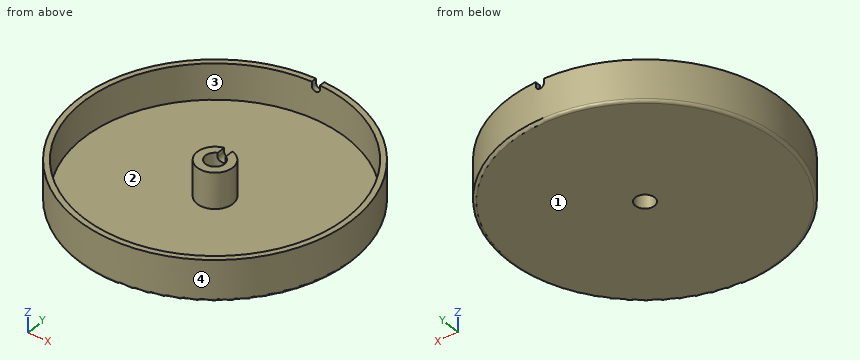
from build123d import *

# Parameters (mm, degrees)
F0_R     = 48
F0_R_2   = 6.5
F1_DEPTH = 2
F0_R_3   = 50
F0_R_4   = 3.5
F2_DEPTH = 15
F4_DEPTH = 70
F5_R     = 1


with BuildPart() as f1:
    # F0 (on Top) → F1 (new body)
    with BuildSketch(Plane.XY):
        Circle(F0_R)
        Circle(F0_R_2, mode=Mode.SUBTRACT)
    extrude(amount=F1_DEPTH)

    # F0 (on Top) → F2 (join)
    with BuildSketch(Plane.XY):
        Circle(F0_R_3)
        Circle(F0_R, mode=Mode.SUBTRACT)
        Circle(F0_R_2)
        Circle(F0_R_4, mode=Mode.SUBTRACT)
    extrude(amount=F2_DEPTH)

    # F3 (on Front) → F4 (cut)
    with BuildSketch(Plane.XZ):
        with BuildLine():
            ThreePointArc((-1.5, 13.5), (0, 15), (1.5, 13.5))
            Line((1.5, 13.5), (1.5, 16.5))
            Line((1.5, 16.5), (-1.5, 16.5))
            Line((-1.5, 16.5), (-1.5, 13.5))
        make_face()
        with BuildLine():
            Line((-1.5, 13.5), (1.5, 13.5))
            ThreePointArc((1.5, 13.5), (0, 15), (-1.5, 13.5))
        make_face()
        with BuildLine():
            ThreePointArc((-1.5, 13.5), (0, 12), (1.5, 13.5))
            Line((1.5, 13.5), (-1.5, 13.5))
        make_face()
    extrude(amount=-F4_DEPTH, mode=Mode.SUBTRACT)

    # F5
    f5_edges = [f1.edges().sort_by_distance(p)[0] for p in [
        (-50, 0, 0),
    ]]
    fillet(f5_edges, radius=F5_R)


solid = f1.part
Read the model definition and answer for the solid it produces. Units are mm, in the model's axes. Face numbers are marked on the shaded views. Coordinates: 2 decimals unless noted, no trailing zeros. Order: outer loops, then holes, each group sorted by start corner. A loop starts at its lowest first (then second) coordinate and runs counter-clockwise, first axis right, second up. Notation, with made-up numbers: M 61,-26.5 L 75,-26.5 A25 ccw 75,12.5 Z; hole C 43.5,-12.5 d1. An arc over 180 degrees is marked long. Put each result on its own line as item: value. Start each with the question number.
Item 1: The mould has two halves that part along Y. Classify the marked faces 1, 2, 3 and 4: +Y half, -Y half, draft (parallel to the pull), parting line (faces both ways), or undercut.
Item 2: Section C-C, the plane z = 10.25 is taken. Determine the outline of the cut face in (x, y).
Item 3: Given pin 1 Ø1.2 at (y, z) = (5, 14.5) entering from +X; pin 2 Ø2 at (x, z) = (14, 12.5) entering from +Y; pin 3 Ø1.5 at (x, y) = (-20.5, -1.5) entering from +Z, each flat-ended and moving along its own axis, determine where each tip first touches the part or whether it passes through.
Item 4: Section A-A, the plane x = 0 is taken. Determine the outline of the cut face in (y, z).
Item 5: Section B-B, the plane y = 0 is taken. Determine the outline of the cut face in (x, z), plus the area to 3 significant figures.
Item 6: Consider probe 1 along X at (y, z) = (0, 3.25); probe 2 along X at (y, z) = (-3, 7.75). Determine where each line is inside the solid, lowest interval first. Write a range as [from, to].
Computed:
1. face 1: draft
1. face 2: undercut
1. face 3: undercut
1. face 4: parting line
2. outline: C 0,0 d100; C 0,0 d13; hole C 0,0 d96; hole C 0,0 d7
3. pin 1: stops at x = 49.81
3. pin 2: stops at y = 48.28
3. pin 3: stops at z = 2
4. outline: M -50,1 A1 ccw -49,0 L -3.5,0 L -3.5,15 L -6.5,15 L -6.5,2 L -48,2 L -48,15 L -50,15 Z; M 3.5,0 L 49,0 A1 ccw 50,1 L 50,12 L 48,12 L 48,2 L 6.5,2 L 6.5,12 L 3.5,12 Z
5. outline: M -50,1 A1 ccw -49,0 L -3.5,0 L -3.5,15 L -6.5,15 L -6.5,2 L -48,2 L -48,15 L -50,15 Z; M 3.5,0 L 49,0 A1 ccw 50,1 L 50,15 L 48,15 L 48,2 L 6.5,2 L 6.5,15 L 3.5,15 Z
5. area: 316 mm2
6. probe 1: x = [-50, -48], [-6.5, -3.5], [3.5, 6.5], [48, 50]
6. probe 2: x = [-49.91, -47.91], [-5.77, -1.8], [1.8, 5.77], [47.91, 49.91]
